Work out the finished part from the listing and answer in its coordinate system (mm). Face numbers are marked on the shaded views. A direction names the side the tool comes from. Round coordinates to 2 decimals unless told otherwise and drop trailing zeros. Write each loop counter-clockwise with the first axis right and the second up, starting at its lowest first coordinate (ties: lowest second). Pieces come first, ordered by that corner, then holes. Notation, with made-up numbers: (65, 51) - (88, 51) arc R21 ccw to (88, 80) - close; hole circle Ø4 at (0, -19.5). An arc over 180 degrees is marked (long way). Answer as a JSON object with one key per item and string values.
```python
from build123d import *

# Parameters (mm, degrees)
SKETCH1_W                                   = 80
SKETCH1_H                                   = 20
BOSS_EXTRUDE1_DEPTH                         = 60
F_2_MM_TOP_BOT_3_MM_SIDE_T                  = -3
F_2_MM_TOP_BOT_3_MM_SIDE_THICKNESS_3_FACE_W = 54
F_2_MM_TOP_BOT_3_MM_SIDE_THICKNESS_3_FACE_H = 17
F_2_MM_TOP_BOT_3_MM_SIDE_THICKNESS_3_DEPTH  = 2
CUT_EXTRUDE1_DEPTH                          = 3
SKETCH4_R                                   = 3.55
CUT_EXTRUDE3_DEPTH                          = 10
F_5_MM_RADIUS_R                             = 5
F_8_5_START                                 = -2
SKETCH7_R                                   = 4.25
F_8_5_MM_HOLD_OFFSET_2_MM_DEPTH             = 3.2


with BuildPart() as part:
    # Sketch1 → Boss-Extrude1 (new body)
    with BuildSketch(Plane(origin=(0, 0, 0), x_dir=(0, 1, 0), z_dir=(0, 0, 1))):
        Rectangle(SKETCH1_W, SKETCH1_H)
    extrude(amount=BOSS_EXTRUDE1_DEPTH)

    # 2 mm top/bot 3 mm side
    f_2_mm_top_bot_3_mm_side_openings = [part.faces().sort_by_distance(p)[0] for p in [
        (-10, 0, 30),
    ]]
    offset(amount=F_2_MM_TOP_BOT_3_MM_SIDE_T, openings=f_2_mm_top_bot_3_mm_side_openings, kind=Kind.INTERSECTION)

    # 2 mm top/bot 3 mm side thickness 3 face (on inner face of the shell) → 2 mm top/bot 3 mm side thickness 3 (add)
    with BuildSketch(Plane(origin=(-1.5, -37, 30), x_dir=(0, 0, -1), z_dir=(0, -1, 0))):
        Rectangle(F_2_MM_TOP_BOT_3_MM_SIDE_THICKNESS_3_FACE_W, F_2_MM_TOP_BOT_3_MM_SIDE_THICKNESS_3_FACE_H)
    extrude(amount=-F_2_MM_TOP_BOT_3_MM_SIDE_THICKNESS_3_DEPTH)

    # Sketch3 → Cut-Extrude1 (cut)
    with BuildSketch(Plane(origin=(0, 0, 0), x_dir=(1, 0, 0), z_dir=(0, 0, -1))):
        with BuildLine():
            ThreePointArc((4.9, 22.5), (3.464823228, 25.964823228), (0, 27.4))
            Line((0, 27.4), (0, 17.6))
            ThreePointArc((0, 17.6), (3.464823228, 19.035176772), (4.9, 22.5))
        make_face()
        with BuildLine():
            Line((0, 17.6), (0, 27.4))
            ThreePointArc((0, 27.4), (-4.9, 22.5), (0, 17.6))
        make_face()
        with BuildLine():
            ThreePointArc((4.9, 7.5), (3.464823228, 10.964823228), (0, 12.4))
            Line((0, 12.4), (0, 2.6))
            ThreePointArc((0, 2.6), (3.464823228, 4.035176772), (4.9, 7.5))
        make_face()
        with BuildLine():
            Line((0, 2.6), (0, 12.4))
            ThreePointArc((0, 12.4), (-4.9, 7.5), (0, 2.6))
        make_face()
        with BuildLine():
            ThreePointArc((4.9, -7.5), (3.464823228, -4.035176772), (0, -2.6))
            Line((0, -2.6), (0, -12.4))
            ThreePointArc((0, -12.4), (3.464823228, -10.964823228), (4.9, -7.5))
        make_face()
        with BuildLine():
            Line((0, -12.4), (0, -2.6))
            ThreePointArc((0, -2.6), (-4.9, -7.5), (0, -12.4))
        make_face()
        with BuildLine():
            ThreePointArc((4.9, -22.5), (3.464823228, -19.035176772), (0, -17.6))
            Line((0, -17.6), (0, -27.4))
            ThreePointArc((0, -27.4), (3.464823228, -25.964823228), (4.9, -22.5))
        make_face()
        with BuildLine():
            Line((0, -27.4), (0, -17.6))
            ThreePointArc((0, -17.6), (-4.9, -22.5), (0, -27.4))
        make_face()
    extrude(amount=-CUT_EXTRUDE1_DEPTH, mode=Mode.SUBTRACT)

    # Sketch4 → Cut-Extrude3 (cut)
    with BuildSketch(Plane.XY.offset(60)):
        with Locations((0, 24.2)):
            Circle(SKETCH4_R)
        Circle(SKETCH4_R)
        with Locations((0, -24.2)):
            Circle(SKETCH4_R)
    extrude(amount=-CUT_EXTRUDE3_DEPTH, mode=Mode.SUBTRACT)

    # 5 mm radius
    f_5_mm_radius_edges = [part.edges().sort_by_distance(p)[0] for p in [
        (7, -35, 30),
        (7, 37, 30),
        (10, -40, 30),
        (10, 40, 30),
    ]]
    fillet(f_5_mm_radius_edges, radius=F_5_MM_RADIUS_R)

    # Sketch7 → 8.5 mm hold offset 2 mm (cut)
    with BuildSketch(Plane(origin=(0, 40, 0), x_dir=(-1, 0, 0), z_dir=(0, 1, 0)).offset(F_8_5_START)):
        with Locations(Location((2.5, 30, 0), (0, 0, 90))):
            Circle(SKETCH7_R)
    f_8_5_mm_hold_offset_2_mm = extrude(amount=-F_8_5_MM_HOLD_OFFSET_2_MM_DEPTH, mode=Mode.SUBTRACT)

    # Mirror1: 8.5 mm hold offset 2 mm across plane
    add(f_8_5_mm_hold_offset_2_mm.mirror(Plane.ZX), mode=Mode.SUBTRACT)


solid = part.part
```
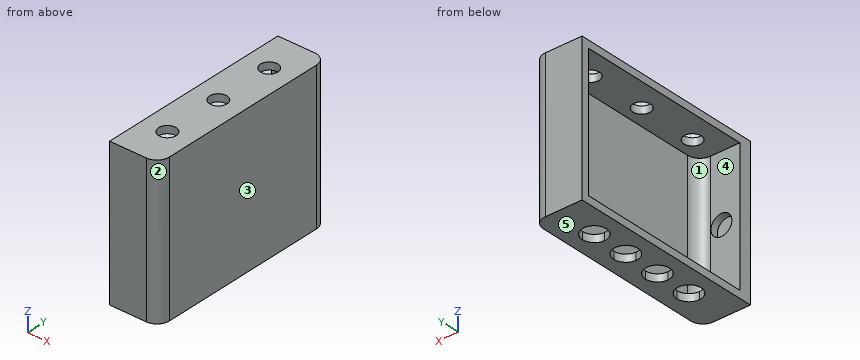
Item 1: Consider line 1 along Y through (x, z) = (-7.25, 38); line 2 along Y through (x, z) = (0, 58.7); line 3 along Z through (x, y) = (6.75, -5.5). Determine where each line is inside the solid, lowest interval first.
Results found:
{"line 1": "-40 to -35, 37 to 40", "line 2": "-40 to -27.75, -20.65 to -3.55, 3.55 to 20.65, 27.75 to 40", "line 3": "0 to 3, 57 to 60"}
Item 2: Each of these flat-tipped pins is pushed along its axis until it touches: P1, Ø6.5, axis at x = 0, y = -24.2, coming from the +Z side; P2, Ø4.5, axis at x = 0, y = 24.2, coming from the -Z side; P3, Ø8, axis at y = -11, z = 50, coming from the -X side; P4, Ø1.5, axis at x = 7, z = 19.5, coming from the +Y side. Where does it stop, or does it pass through?
Results found:
{"P1": "z = 3", "P2": "through", "P3": "x = 7", "P4": "y = 39.84"}
Item 3: A cutting plane is placed at D-D (x = -1.25). Give the number of separate pieces and of enclosed holes in the cut face, and give its area (3 significant figures).
Results found:
{"separate pieces": "7", "enclosed holes": "0", "area": "706 mm²"}
Item 4: A cutting plane is placed at A-A (y = -5). Write down the section's boundary in (x, z).
Results found:
{"outline": "(-10, 0) - (-4.21, 0) - (-4.21, 3) - (-10, 3) - close; (-10, 57) - (7, 57) - (7, 3) - (4.21, 3) - (4.21, 0) - (10, 0) - (10, 60) - (-10, 60) - close"}
Item 5: A cutting plane is placed at B-B (z = 18). Write down the section's boundary in (x, y), and give its area (3 significant figures).
Results found:
{"outline": "(-10, -40) - (5, -40) arc R5 ccw to (10, -35) - (10, 35) arc R5 ccw to (5, 40) - (-10, 40) - (-10, 37) - (2, 37) arc R5 cw to (7, 32) - (7, -30) arc R5 cw to (2, -35) - (-10, -35) - close", "area": "376 mm²"}
Item 6: Determine the mould class of the marked faces 3, 4 and 5 for opening direction Z: pulls with the +Z half, pulls with the -Z half, needs draft (parallel to the pull), parting line crosses it, or undercut.
Results found:
{"face 3": "needs draft", "face 4": "undercut", "face 5": "pulls with the -Z half"}
Item 7: For the marked faces 1 and 2, determine the directions among +Z, -Z, +X, -X, +Y, -Y from which every point of the face is accessible in a straight line to the end or side of a thin tool.
Results found:
{"face 1": "-X", "face 2": "+Z, -Z, +X, -Y"}
Item 8: A cutting plane is placed at C-C (y = -24.2). Write down the section's boundary in (x, z), and give its area (3 significant figures).
Results found:
{"outline": "(-10, 0) - (-4.6, 0) - (-4.6, 3) - (-10, 3) - close; (-10, 57) - (-3.55, 57) - (-3.55, 60) - (-10, 60) - close; (3.55, 57) - (7, 57) - (7, 3) - (4.6, 3) - (4.6, 0) - (10, 0) - (10, 60) - (3.55, 60) - close", "area": "233 mm²"}
